Could you check a few things on this model? Use its own coordinates, in mm. Face numbers are marked on the shaded views. Give positions to 0.01 mm unless a question says otherwise; leave off trailing zeros. Order: outer loops, then holes, each group sorted by start corner. A loop starts at its lowest first (then second) coordinate and runs counter-clockwise, first axis right, second up. Notation, with made-up numbers: M 5.5,27.5 L 30.5,27.5 A7 ccw 30.5,40.5 Z; hole C 1,-34 d3. An arc over 180 degrees is marked long. Use a Markdown table: item, result. Add a question column.
Item 1: I'm going to push flat-ended pins straight in: pin 1 Ø1 at (y, z) = (9.5, -14.5) entering from +X; pin 2 Ø2 at (y, z) = (7, -12.5) entering from +X; pin 3 Ø2 at (y, z) = (27, -3.5) entering from -X. Where does each tip first touch, or does it pass through?
Item 2: Suppose I cut it at C-C on x = 7. Write out the boundary of the cut face in (y, z), plus the area to 3 significant figures.
Item 3: If we mould it in two halves opening along X, with no side actions, what happens to the marked faces 1, 2 and 3? For each: released by +X, released by -X, zero draft, split by the parting line, or undercut.
Item 4: If I drill on L1, parallel to X at y = 22.5, z = -8; L2, parallel to Y at x = 7, z = -6.75; L3, parallel to X at y = 21, z = -8, over which ranges is the centre line in solid material (lowest first)? Write a range as from..to.
Item 5: Suppose I cut it at D-D on y = 14. Write out the boundary of the cut face in (x, z), plus the area to 3 significant figures.
Item 6: Suppose I cut it at B-B on y = 20. Write out the boundary of the cut face in (x, z), plus the area to 3 significant figures.
Item 7: Suppose I cut it at A-A on z = -8. Write out the boundary of the cut face in (x, y).
from build123d import *

# Parameters (mm, degrees)
SKETCH1_W           = 50
SKETCH1_H           = 16
SKETCH1_R           = 1.6
BOSS_EXTRUDE1_DEPTH = 40
SKETCH2_R           = 1.6
CUT_EXTRUDE1_DEPTH  = 67
FILLET1_R           = 5


with BuildPart() as part:
    # Sketch1 → Boss-Extrude1 (new body)
    with BuildSketch(Plane(origin=(0, 0, 0), x_dir=(1, 0, 0), z_dir=(0, 1, 0))):
        with Locations((25, 8)):
            Rectangle(SKETCH1_W, SKETCH1_H)
        with Locations(Location((15, 8, 0), (0, 0, 270))):
            Circle(SKETCH1_R, mode=Mode.SUBTRACT)
        with Locations(Location((35, 8, 0), (0, 0, 270))):
            Circle(SKETCH1_R, mode=Mode.SUBTRACT)
    extrude(amount=BOSS_EXTRUDE1_DEPTH)

    # Sketch2 → Cut-Extrude1 (cut, through all)
    with BuildSketch(Plane.XY):
        with Locations((7, 20)):
            Circle(SKETCH2_R)
        with Locations((43, 20)):
            Circle(SKETCH2_R)
    extrude(amount=-CUT_EXTRUDE1_DEPTH, mode=Mode.SUBTRACT)

    # Fillet1
    fillet1_edges = [part.edges().sort_by_distance(p)[0] for p in [
        (0, 20, -16),
        (50, 20, -16),
        (50, 20, 0),
        (0, 20, 0),
    ]]
    fillet(fillet1_edges, radius=FILLET1_R)


solid = part.part
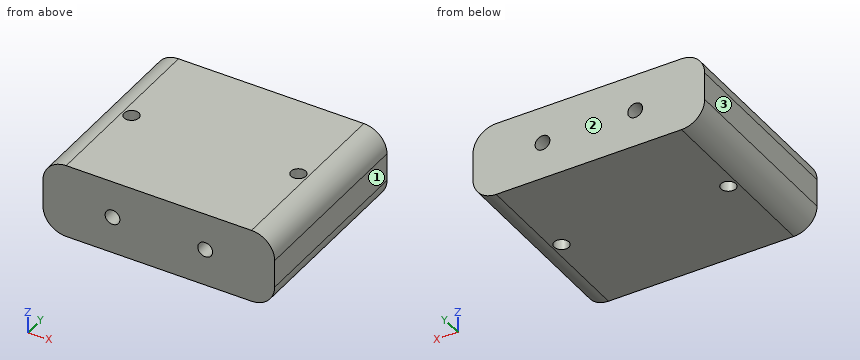
Findings below:
| question | item | result |
|---|---|---|
| 1 | pin 1 | stops at x = 49 |
| 1 | pin 2 | stops at x = 49.97 |
| 1 | pin 3 | stops at x = 0.03 |
| 2 | outline | M 0,-16 L 18.4,-16 L 18.4,0 L 0,0 Z; M 21.6,-16 L 40,-16 L 40,0 L 21.6,0 Z |
| 2 | area | 589 mm^2 |
| 3 | face 1 | released by +X |
| 3 | face 2 | zero draft |
| 3 | face 3 | released by -X |
| 4 | L1 | x = 0..13.4, 16.6..33.4, 36.6..50 |
| 4 | L2 | y = 0..18.4, 21.6..40 |
| 4 | L3 | x = 0..5.75, 8.25..13.4, 16.6..33.4, 36.6..41.75, 44.25..50 |
| 5 | outline | M 0,-11 A5 ccw 5,-16 L 45,-16 A5 ccw 50,-11 L 50,-5 A5 ccw 45,0 L 5,0 A5 ccw 0,-5 Z; hole C 15,-8 d3.2; hole C 35,-8 d3.2 |
| 5 | area | 762 mm^2 |
| 6 | outline | M 0,-11 A5 ccw 5,-16 L 5.4,-16 L 5.4,0 L 5,0 A5 ccw 0,-5 Z; M 8.6,-16 L 41.4,-16 L 41.4,0 L 8.6,0 Z; M 44.6,-16 L 45,-16 A5 ccw 50,-11 L 50,-5 A5 ccw 45,0 L 44.6,0 Z; hole C 15,-8 d3.2; hole C 35,-8 d3.2 |
| 6 | area | 660 mm^2 |
| 7 | outline | M 0,0 L 13.4,0 L 13.4,40 L 0,40 Z; M 16.6,0 L 33.4,0 L 33.4,40 L 16.6,40 Z; M 36.6,0 L 50,0 L 50,40 L 36.6,40 Z; hole C 7,20 d3.2; hole C 43,20 d3.2 |
